Design review of the part built by this model. Coordinates are the model's own, in mm. Coordinates: 2 decimals unless noted, no trailing zeros. Loops run counter-clockwise (first coordinate to the right, second up) from the corner with the lowest first, then second, coordinate; pieces in that order, holes last.
Autodesk Inventor part; units mm, degrees
ref_plane "YZ Plane" through (0, 0, 0) normal (1, 0, 0) x (0, 1, 0)
ref_plane "XZ Plane" through (0, 0, 0) normal (0, 1, 0) x (-1, 0, 0)
ref_plane "XY Plane" through (0, 0, 0) normal (0, 0, 1) x (1, 0, 0)
sketch "Эскиз1" plane through (0, 0, 0) normal (0, 0, 1) x (1, 0, 0)
  line L0 (4, 0) -> (50, 0)
  line L1 (70, -4) -> (70, -49)
  line L2 (66, -65) -> (4, -65)
  line L3 (0, -61) -> (0, -4)
  arc A0 (70, -4) -> (66, 0) centre (66, -4) ccw
  arc A1 (66, -65) -> (70, -61) centre (66, -61) ccw
  arc A2 (4, 0) -> (0, -4) centre (4, -4) ccw
  arc A3 (0, -61) -> (4, -65) centre (4, -61) ccw
  line L4 (-10, 25) -> (50, 25)
  line L5 (65, 25) -> (65, -25)
  line L6 (65, -25) -> (-10, -25)
  line L7 (-10, -25) -> (-10, 25)
  line L8 (-10, 25) -> (65, -25) construction
  line L9 (65, 25) -> (-10, -25) construction
  line L10 (70, -49) -> (50, -49)
  line L11 (50, -49) -> (50, 25)
  line L12 (70, -49) -> (70, -61)
  line L13 (65, 0) -> (66, 0)
  line L14 (50, 0) -> (65, 0)
  line L15 (50, 25) -> (65, 25)
  point P0 (0, 0)
  point P1 (70, -65)
  point P2 (70, 0)
  point P3 (27.5, 0)
  point P4 (5, 0)
  point P5 (65, 0)
  point P6 (50, -25)
  point P7 (0, -25)
  dimension "d0" = 70
  dimension "d1" = 65
  dimension "d2" = 4
  dimension "d23" = 75
  dimension "d24" = 50
  dimension "d44" = 20
  dimension "d46" = 16
  dimension "d47" = 5
  dimension "d48" = 25
extrude "Выдавливание1" add sketch "Эскиз1" along normal blind 4 contours A2 L3 L6 L7 L4 L11 L0 | L0 L11 L6 L3 A2 | L11 L10 L12 A1 L2 A3 L3 L6
sketch "Эскиз2" plane through (0, 0, 4) normal (0, 0, 1) x (1, 0, 0)
  circle A0 centre (61, -57) radius 3.5
  line L0 (4, -65) -> (66, -65)
  circle A1 centre (8, -57) radius 3.5
  line L1 (0, -25) -> (0, -61)
  circle A2 centre (61, -17) radius 3.5
  circle A3 centre (8, -17) radius 3.5
  line L2 (61, -17) -> (8, -17) construction
  line L3 (61, -17) -> (61, -57) construction
  line L4 (8, -57) -> (61, -57)
  circle A4 centre (54.5, 12) radius 2.5
  line L5 (54.5, 12) -> (54.5, -22.1685) construction
  circle A5 centre (2, 12) radius 2.5
  line L6 (70, -61) -> (70, -49)
  line L7 (-10, 25) -> (-10, -25)
  dimension "d5" = 7
  dimension "d6" = 8
  dimension "d8" = 7
  dimension "d9" = 8
  dimension "d10" = 8
  dimension "d13" = 7
  dimension "d16" = 7
  dimension "d19" = 53
  dimension "d20" = 53
  dimension "d21" = 40
  dimension "d22" = 40
  dimension "d26" = 5
  dimension "d27" = 29
  dimension "d28" = 6.5
  dimension "d29" = 5
  dimension "d43" = 29
  dimension "d51" = 12
extrude "Выдавливание2" cut sketch "Эскиз2" against normal blind 4
fillet "Сопряжение1" radius 4 1 edges at (-10, 25, 2)
sketch "Эскиз3" plane through (0, 0, 4) normal (0, 0, 1) x (1, 0, 0)
  circle A0 centre (2, 12) radius 2.5 construction
  line L0 (67, 12) -> (2, 12) construction
  line L1 (34.5, 12) -> (34.5, -39.6855) construction
  circle A1 centre (34.5, 12) radius 2
  circle A2 centre (34.5, -3) radius 2
  circle A3 centre (34.5, -18) radius 2
  line L2 (50, -49) -> (50, 25)
  point P0 (0, 0)
  dimension "d31" = 4
  dimension "d32" = 4
  dimension "d33" = 4
  dimension "d34" = 15
  dimension "d35" = 15
  dimension "d50" = 15.5
extrude "Выдавливание3" cut sketch "Эскиз3" against normal blind 10
fillet "Сопряжение3" radius 4 3 edges at (50, 25, 2) (50, -49, 2) (70, -49, 2)
sketch "Эскиз5" plane through (0, 0, 4) normal (0, 0, 1) x (1, 0, 0)
  circle A0 centre (79.889, -5.5) radius 8 construction
  line L0 (79.889, 2.5) -> (-3.7783, 2.5) construction
  point P0 (0, 0)
fillet "Сопряжение4" radius 4 2 edges at (0, -25, 2) (-10, -25, 2)
properties part number "креп_центр_рейки"
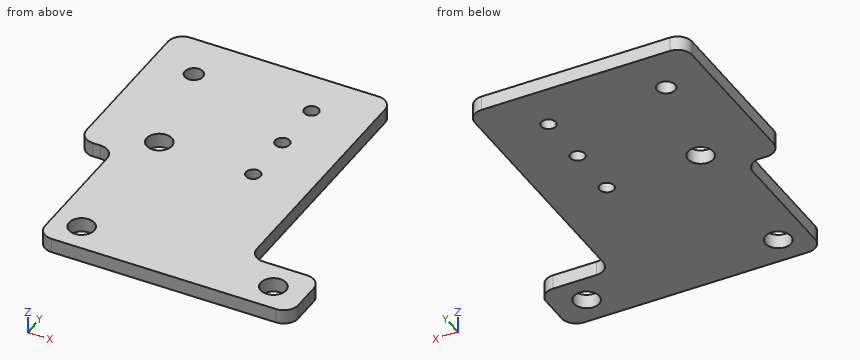
Q1. Take a section at B-B, the plane y = -57. Write out the cut boundary in (x, z).
Q2. Take a section at D-D, the plane z = 2.6. Write out the cut boundary in (x, y).
Q3. Clearance check with flat-ended pins moving along their axes: pin 1 Ø2 at (y, z) = (-37, 2.5) entering from -X; pin 2 Ø1.2 at (y, z) = (1, 2.5) entering from +X; pin 3 Ø1.5 at (y, z) = (-28, 2.5) entering from -X. State where each tip first meets the part, or that it passes through.
Q4. Take a section at C-C, the plane x = 34.5. Write out the cut boundary in (y, z), then the cut area to 3 significant figures.
Q5. For line 1 (Y direction, x = 34.5, z = 2.9); line 2 (Y direction, x = 8, z = 1.15); line 3 (Y direction, x = 9, z = 2.8), list the stretches that pass through material, from the lowest coordinate up.
Q6. Take a section at A-A, the plane x = 61. Write out the cut boundary in (y, z), then the cut area to 3 significant figures.
Entries:
1. outline: (0, 0) - (4.5, 0) - (4.5, 4) - (0, 4) - close; (11.5, 0) - (57.5, 0) - (57.5, 4) - (11.5, 4) - close; (64.5, 0) - (70, 0) - (70, 4) - (64.5, 4) - close
2. outline: (-10, -21) arc R4 ccw to (-6, -25) - (-4, -25) arc R4 cw to (0, -29) - (0, -61) arc R4 ccw to (4, -65) - (66, -65) arc R4 ccw to (70, -61) - (70, -53) arc R4 ccw to (66, -49) - (54, -49) arc R4 cw to (50, -45) - (50, 21) arc R4 ccw to (46, 25) - (-6, 25) arc R4 ccw to (-10, 21) - close; hole circle Ø5 at (2, 12); hole circle Ø7 at (8, -57); hole circle Ø7 at (8, -17); hole circle Ø4 at (34.5, -18); hole circle Ø4 at (34.5, -3); hole circle Ø4 at (34.5, 12); hole circle Ø7 at (61, -57)
3. pin 1: stops at x = 0
3. pin 2: stops at x = 50
3. pin 3: stops at x = -0.4
4. outline: (-65, 0) - (-20, 0) - (-20, 4) - (-65, 4) - close; (-16, 0) - (-5, 0) - (-5, 4) - (-16, 4) - close; (-1, 0) - (10, 0) - (10, 4) - (-1, 4) - close; (14, 0) - (25, 0) - (25, 4) - (14, 4) - close
4. area: 312 mm2
5. line 1: y = -65 to -20, -16 to -5, -1 to 10, 14 to 25
5. line 2: y = -65 to -60.5, -53.5 to -20.5, -13.5 to 25
5. line 3: y = -65 to -60.35, -53.65 to -20.35, -13.65 to 25
6. outline: (-65, 0) - (-60.5, 0) - (-60.5, 4) - (-65, 4) - close; (-53.5, 0) - (-49, 0) - (-49, 4) - (-53.5, 4) - close
6. area: 36.0 mm2
